Can you work these out from the model? Positions are in its coordinate system, mm. A direction names the side the tool comes from. Give positions to 0.01 mm unless a question says otherwise; leave off trailing zeros. Write each loop counter-clockwise with the first axis right and the second up, starting at its lowest first coordinate (ties: lowest second). Pieces come first, ordered by that corner, then holes. Notation, with made-up numbers: (87, 70) - (120, 70) arc R12 ccw to (120, 82) - close; hole circle Ø3 at (40.25, -33). An arc over 180 degrees is marked (long way). Use a Markdown table: item, result. Add a question column.
Autodesk Inventor part; units mm, degrees
ref_plane "YZ Plane" through (0, 0, 0) normal (1, 0, 0) x (0, 1, 0)
ref_plane "XZ Plane" through (0, 0, 0) normal (0, 1, 0) x (-1, 0, 0)
ref_plane "XY Plane" through (0, 0, 0) normal (0, 0, 1) x (1, 0, 0)
sketch "Sketch1" plane through (0, 0, 0) normal (0, 0, 1) x (1, 0, 0)
  arc A0 (-4, 0) -> (4, 0) centre (0, 0) ccw
  line L0 (-4, 0) -> (-12.5, 0)
  line L1 (-12.5, 0) -> (-12.5, -10)
  line L2 (-12.5, -10) -> (12.5, -10)
  line L3 (12.5, -10) -> (12.5, 0)
  line L4 (12.5, 0) -> (4, 0)
  dimension "d0" = 4
  dimension "d1" = 10
  dimension "d2" = 25
extrude "Extrusion1" add sketch "Sketch1" along normal blind 6
sketch "Sketch2" plane through (-12.5, 0, 0) normal (0, 1, 0) x (1, 0, 0)
  line L0 (0, 0) -> (8.5, 0)
  line L1 (8.5, -6) -> (0, -6)
  line L2 (16.5, 0) -> (25, 0)
  line L3 (16.5, 0) -> (16.5, -6)
  line L4 (25, -6) -> (16.5, -6)
  line L5 (25, 0) -> (25, -6)
  line L6 (4.25, 0) -> (4.25, -6) construction
  line L7 (20.75, 0) -> (20.75, -6) construction
  circle A0 centre (4.25, -3) radius 1.75
  circle A1 centre (20.75, -3) radius 1.75
  point P0 (12.5, 0)
  dimension "d5" = 3.5
extrude "Extrusion2" cut sketch "Sketch2" against normal through all contours A0 | A1
sketch "Sketch3" plane through (0, 0, 6) normal (0, 0, 1) x (1, 0, 0)
  line L0 (12.5, -10) -> (12.5, 0)
  line L1 (-12.5, 0) -> (12.5, 0)
  line L2 (12.5, 0) -> (12.5, -1)
  line L3 (12.5, -1) -> (-12.5, -1)
  line L4 (-12.5, -1) -> (-12.5, 0)
  dimension "d8" = 1
extrude "Extrusion3" cut sketch "Sketch3" against normal through all
sketch "Sketch4" plane through (0, 0, 6) normal (0, 0, 1) x (1, 0, 0)
  line L0 (4.7625, -4.7625) -> (-4.7625, -4.7625)
  line L1 (-4.7625, -4.7625) -> (-4.7625, 4.7625)
  line L2 (-4.7625, 4.7625) -> (4.7625, 4.7625)
  line L3 (4.7625, 4.7625) -> (4.7625, -4.7625)
  line L4 (4.7625, -4.7625) -> (-4.7625, 4.7625) construction
  line L5 (-4.7625, -4.7625) -> (4.7625, 4.7625) construction
  point P0 (0, 0)
  dimension "d11" = 9.525
extrude "Extrusion4" cut sketch "Sketch4" against normal through all
properties part number "sensor bracket coupler"
Q1. If we mould it in two halves opening along Z, with no side actions, what happens to faces 1 (the flat face through (0, -5, 6)), 2 (the flat face through (-10.3, -1, 3)), 3 (the cylindrical face through (9.867, -5.437, 3.67))? For each: released by +Z, released by -Z, zero draft, split by the parting line, or undercut.
Q2. Suppose I cut it at B-B (x = -8.25). Please give me the cut outline in (y, z), and give its area (3 significant figures).
Q3. Suppose I cut it at D-D (y = -9). Please give me the cut outline in (x, z), and give its area (3 significant figures).
Q4. If I drill on probe 1 along X at (y, z) = (-6, 3); probe 2 along X at (y, z) = (-3, 3); probe 3 along X at (y, z) = (-1.75, 5), over which ranges is the centre line in solid material (lowest first)? Write a range as [from, to].
Q5. On a 3-axis mill with a long thin cutter (end or side, diameter ignored), from which of +Z, -Z, +X, -X, +Y, -Y can I reach the whole of each face in a straight line? I mean faces 4 (the flat face through (10, -1, 4)), 5 (the flat face through (-4.762, -3, 3)). Say none if no direction works.
Q6. Suppose I cut it at A-A (y = -1.25). Please give me the cut outline in (x, z), and give its area (3 significant figures).
Q7. Suppose I cut it at C-C (z = 3). Please give me the cut outline in (x, y), and give its area (3 significant figures).
Q8. I'm going to push a flat-ended pin straight in: P1, Ø3, axis at x = -8.25, z = 3, coming from the -Y side. Where does the tip first touch, or does it pass through?
Derived:
| question | item | result |
|---|---|---|
| 1 | face 1 | released by +Z |
| 1 | face 2 | zero draft |
| 1 | face 3 | undercut |
| 2 | outline | (-10, 0) - (-1, 0) - (-1, 1.25) - (-10, 1.25) - close; (-10, 4.75) - (-1, 4.75) - (-1, 6) - (-10, 6) - close |
| 2 | area | 22.5 mm² |
| 3 | outline | (-12.5, 0) - (12.5, 0) - (12.5, 6) - (-12.5, 6) - close; hole circle Ø3.5 at (-8.25, 3); hole circle Ø3.5 at (8.25, 3) |
| 3 | area | 131 mm² |
| 4 | probe 1 | [-12.5, -10], [-6.5, 6.5], [10, 12.5] |
| 4 | probe 2 | [-12.5, -10], [-6.5, -4.76], [4.76, 6.5], [10, 12.5] |
| 4 | probe 3 | [-12.5, -4.76], [4.76, 12.5] |
| 5 | face 4 | +Z, -Z, +X, -X, +Y |
| 5 | face 5 | +Z, -Z, +Y |
| 6 | outline | (-12.5, 0) - (-4.76, 0) - (-4.76, 6) - (-12.5, 6) - close; (4.76, 0) - (12.5, 0) - (12.5, 6) - (4.76, 6) - close; hole circle Ø3.5 at (-8.25, 3); hole circle Ø3.5 at (8.25, 3) |
| 6 | area | 73.6 mm² |
| 7 | outline | (-12.5, -10) - (-10, -10) - (-10, -1) - (-12.5, -1) - close; (-6.5, -10) - (6.5, -10) - (6.5, -1) - (4.76, -1) - (4.76, -4.76) - (-4.76, -4.76) - (-4.76, -1) - (-6.5, -1) - close; (10, -10) - (12.5, -10) - (12.5, -1) - (10, -1) - close |
| 7 | area | 126 mm² |
| 8 | P1 | through |
